Autodesk Inventor part; units mm, degrees
ref_plane "YZ Plane" through (0, 0, 0) normal (1, 0, 0) x (0, 1, 0)
ref_plane "XZ Plane" through (0, 0, 0) normal (0, 1, 0) x (-1, 0, 0)
ref_plane "XY Plane" through (0, 0, 0) normal (0, 0, 1) x (1, 0, 0)
sketch "Skizze1" plane through (0, 0, 0) normal (0, 0, 1) x (1, 0, 0)
  line L0 (0, 5) -> (0, 95)
  line L1 (5, 100) -> (45, 100)
  line L2 (50, 95) -> (50, 5)
  arc A0 (5, 100) -> (0, 95) centre (5, 95) ccw
  arc A1 (50, 95) -> (45, 100) centre (45, 95) ccw
  arc A2 (45, 0) -> (50, 5) centre (45, 5) ccw
  arc A3 (0, 5) -> (5, 0) centre (5, 5) ccw
  line L3 (10, 0) -> (10, -11)
  line L4 (10, -11) -> (20, -11)
  line L5 (20, -11) -> (20, 0)
  line L6 (30, 0) -> (30, -11)
  line L7 (30, -11) -> (40, -11)
  line L8 (40, -11) -> (40, 0)
  line L9 (5, 0) -> (10, 0)
  line L10 (20, 0) -> (30, 0)
  line L11 (40, 0) -> (45, 0)
  line L12 (14.3404, 40) -> (14.8102, 39.829)
  line L13 (14.8102, 39.829) -> (7.9698, 21.0351)
  line L14 (7.9698, 21.0351) -> (7.5, 21.2061)
  line L15 (7.5, 21.2061) -> (14.3404, 40)
  line L16 (19.6299, 32.4397) -> (20.0998, 32.2687)
  line L17 (20.0998, 32.2687) -> (13.2594, 13.4748)
  line L18 (13.2594, 13.4748) -> (12.7895, 13.6459)
  line L19 (12.7895, 13.6459) -> (19.6299, 32.4397)
  line L20 (29.5432, 40) -> (30.013, 39.829)
  line L21 (30.013, 39.829) -> (23.1726, 21.0351)
  line L22 (22.7028, 21.2061) -> (29.5432, 40)
  line L23 (23.1726, 21.0351) -> (22.7028, 21.2061)
  line L24 (42.3412, 40) -> (42.8111, 39.829)
  line L25 (35.5008, 21.2061) -> (42.3412, 40)
  line L26 (42.8111, 39.829) -> (35.9707, 21.0351)
  line L27 (35.9707, 21.0351) -> (35.5008, 21.2061)
  line L28 (31.9383, 28.9336) -> (32.4081, 28.7626)
  line L29 (25.0979, 10.1397) -> (31.9383, 28.9336)
  line L30 (32.4081, 28.7626) -> (25.5677, 9.9687)
  line L31 (25.5677, 9.9687) -> (25.0979, 10.1397)
  point P0 (0, 0)
  dimension "d1" = 50
  dimension "d3" = 5
  dimension "d4" = 11
  dimension "d5" = 10
  dimension "d6" = 100
  dimension "d9" = 0.5
  dimension "d10" = 20
  dimension "d11" = 20
  dimension "d12" = 7.5
  dimension "d14" = 40
extrude "Extrusion1" add sketch "Skizze1" along normal blind 3
properties part number "Scheibe" material "Glas"
CAD build for the part. Positions are in the model's coordinates, mm. A direction names the side the tool comes from. Round coordinates to 2 decimals unless told otherwise and drop trailing zeros. Loops run counter-clockwise (first coordinate to the right, second up) from the corner with the lowest first, then second, coordinate; pieces in that order, holes last. Notation, with made-up numbers: M 44,45 L 61,45 A25 cw 61,72 Z; hole C 6,78 d4. An arc over 180 degrees is marked long. One line per question, with ' | ' between items. Start each with the question number.
Item 1: Which spindle directions (+Z, -Z, +X, -X, +Y, -Y) get a long thin tool onto all of the face, cutting with end or side? Do faces 4 (the flat face through (7, 0, 1)), 5 (the flat face through (28.47, 19.41, 1.48)), 6 (the flat face through (25, 0, 1)). Say none if no direction does.
Item 2: Cut at A-A, the plane y = -1. Write the cut outline in (x, z).
Item 3: Cut at C-C, the plane y = 30. Write the cut outline in (x, z).
Item 4: Pin check, flat tips, straight feed: pin 1 Ø1.5 at (y, z) = (-5.5, 2) entering from -X; pin 2 Ø0.9 at (y, z) = (-8, 1) entering from +X; pin 3 Ø1.5 at (x, z) = (23, 1.5) entering from -Y. Stop position of each tip, or through.
Item 5: Two-plate mould, pull along X, no slides. Class faces 1 (the flat face through (42, 0, 1)), 2 (the flat face through (26.075, 30.471, 1.479)), 3 (the flat face through (50, 51, 1)): pulls with the +X half, pulls with the -X half, needs draft (parallel to the pull), parting line crosses it, or undercut.
Item 6: Cut at B-B, the plane x = 27. Write the cut outline in (y, z).
Item 7: Cut at D-D, the plane y = 18. Write the cut outline in (x, z).
Item 8: Wall check: line 1 (X direction, y = 22, z = 1.15); line 2 (X direction, y = 33, z = 2.7); line 3 (X direction, y = 15, z = 2.8). Give the ranges that are in metal, low to high.
Responses:
1) face 4: +Z, -Z, -X, -Y | face 5: +Z, -Z | face 6: +Z, -Z, -Y
2) outline: M 10,0 L 20,0 L 20,3 L 10,3 Z; M 30,0 L 40,0 L 40,3 L 30,3 Z
3) outline: M 0,0 L 10.7,0 L 10.7,3 L 0,3 Z; M 11.23,0 L 18.74,0 L 18.74,3 L 11.23,3 Z; M 19.27,0 L 25.9,0 L 25.9,3 L 19.27,3 Z; M 26.44,0 L 38.7,0 L 38.7,3 L 26.44,3 Z; M 39.23,0 L 50,0 L 50,3 L 39.23,3 Z
4) pin 1: stops at x = 10 | pin 2: stops at x = 40 | pin 3: stops at y = 0
5) face 1: needs draft | face 2: undercut | face 3: pulls with the +X half
6) outline: M 0,0 L 13.9,0 L 13.9,3 L 0,3 Z; M 15.37,0 L 31.55,0 L 31.55,3 L 15.37,3 Z; M 33.01,0 L 100,0 L 100,3 L 33.01,3 Z
7) outline: M 0,0 L 14.37,0 L 14.37,3 L 0,3 Z; M 14.91,0 L 27.96,0 L 27.96,3 L 14.91,3 Z; M 28.49,0 L 50,0 L 50,3 L 28.49,3 Z
8) line 1: x = 0 to 7.79, 8.32 to 15.83, 16.36 to 22.99, 23.52 to 29.41, 29.95 to 35.79, 36.32 to 50 | line 2: x = 0 to 11.79, 12.32 to 27, 27.53 to 39.79, 40.33 to 50 | line 3: x = 0 to 13.28, 13.81 to 26.87, 27.4 to 50
